Check sheet for the modelled part. Datum: model origin and axes. Units: mm. Face numbers are marked on the shaded views. Give positions to 0.01 mm unless a question says otherwise; leave off trailing zeros. Write each loop counter-clockwise with the first axis right and the second up, starting at its lowest first coordinate (ties: lowest second). Pieces come first, ordered by that corner, then holes. Notation, with made-up numbers: M -33,83.5 L -7,83.5 A24 cw -7,119.5 Z; hole C -10.5,11.25 d10. An arc over 180 degrees is marked long. Write item = value, one per line. Start each with the question number.
1) Draft check along Z on the marked faces 1, 2 and 3. Enter one of: pulls with the +Z half, pulls with the -Z half, needs draft (parallel to the pull), parting line crosses it, or undercut.
2) Sectioned sample at B-B, the plane y = 3.5. Record the cut outline in (x, z), then the cut area to 3 significant figures.
3) Scan lines: L1, parallel to X at y = 0.5, z = 0; L2, parallel to X at y = 3.5, z = 0.25. Record each from-to range of solid material in increasing order.
4) Sectioned sample at A-A, the plane y = 1.75. Record the cut outline in (x, z).
5) Gauge pin test, flat ends, axial feed: pin 1 (3 mm diameter, centred on y = -1, z = -4, fed in from -X); pin 2 (3 mm diameter, centred on x = 0, z = 0, fed in from -Y). Record the tip position at first contact, or that the pin passes through.
Solid Edge part; units mm, degrees
sketch "Sketch1" plane through (0, 0, 0) normal (0, -1, 0) x (1, 0, 0)
  line L0 (5, 2.8868) -> (0, 5.7735)
  line L1 (0, 5.7735) -> (-5, 2.8868)
  line L2 (-5, 2.8868) -> (-5, -2.8868)
  line L3 (-5, -2.8868) -> (0, -5.7735)
  line L4 (0, -5.7735) -> (5, -2.8868)
  line L5 (5, -2.8868) -> (5, 2.8868)
extrude "Protrusion1" add sketch "Sketch1" along normal mid plane 4.9
sketch "Sketch2" plane through (0, 0, 0) normal (1, 0, 0) x (0, 1, 0)
  line L0 (-2.45, 5) -> (-2.2427, 5.7735)
revolve "RevolvedCutout1" cut sketch "Sketch2" angle 360 about axis through (0, 0, 0) along (0, -1, 0) material side at (0, -2.3946, 5.3997)
mirror "Mirror1" about plane through (0, 0, 0) normal (0, -1, 0) of "RevolvedCutout1"
sketch "Sketch3" plane through (0, 2.45, 0) normal (0, 1, 0) x (0, 0, -1)
  circle A0 centre (0, 0) radius 5
extrude "Protrusion2" add sketch "Sketch3" along normal blind 3.1
fillet "倒圆_2" radius 0.5 1 edges at (0, 5.55, 5)
hole "孔_7" at (0, -2.45, 0) direction (0, 1, 0) diameter 4.917 end up to next start chamfer 0.6 start chamfer angle 60 end chamfer 0.6 end chamfer angle 60
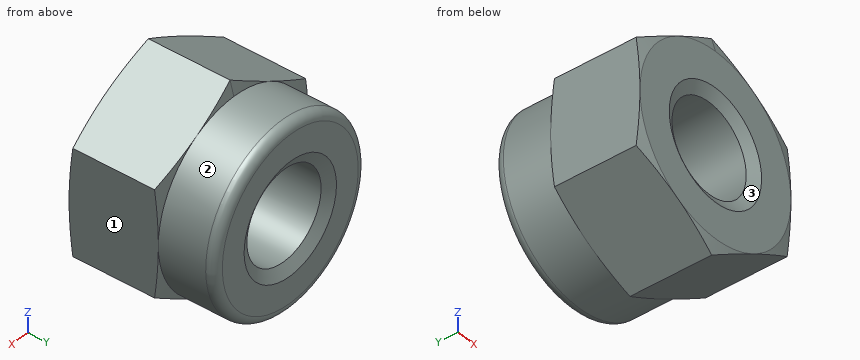
Data:
q1.face_1 = needs draft
q1.face_2 = parting line crosses it
q1.face_3 = undercut
q2.outline = C 0,0 d10; hole C 0,0 d4.92
q2.area = 59.6 mm2
q3.L1 = -5 to -2.46, 2.46 to 5
q3.L2 = -4.99 to -2.45, 2.45 to 4.99
q4.outline = M -5,-2.89 L 0,-5.77 L 5,-2.89 L 5,2.89 L 0,5.77 L -5,2.89 Z; hole C 0,0 d4.92
q5.pin_1 = -5
q5.pin_2 = through
